from build123d import *

# Parameters (mm, degrees)
F0_R     = 4
F1_DEPTH = 3


with BuildPart() as f1:
    # F0 (on Front) → F1 (new body)
    with BuildSketch(Plane.XZ):
        with BuildLine():
            Line((53.104726, 7.336025), (-11.265956, 21.021994))
            ThreePointArc((-11.265956, 21.021994), (-14.82391, 21.160881), (-18.044949, 19.643238))
            Line((-18.044949, 19.643238), (-35.312375, 5.680292))
            ThreePointArc((-35.312375, 5.680292), (-37.891192, -0.597124), (-34.34867, -6.385628))
            Line((-34.34867, -6.385628), (-13.478804, -16.153186))
            ThreePointArc((-13.478804, -16.153186), (-11.393882, -16.717558), (-9.234581, -16.664338))
            Line((-9.234581, -16.664338), (52.653274, -7.417663))
            ThreePointArc((52.653274, -7.417663), (59.041491, -0.229387), (53.104726, 7.336025))
        make_face()
        with Locations((-30.415, 0)):
            Circle(F0_R, mode=Mode.SUBTRACT)
        with BuildLine():
            ThreePointArc((-15.273344, 12.239736), (-14.900729, 15.75558), (-11.384885, 15.382966))
            ThreePointArc((-11.384885, 15.382966), (-6.127117, 2.979875), (-8.230613, -10.326369))
            ThreePointArc((-8.230613, -10.326369), (-11.552104, -11.537854), (-12.76359, -8.216363))
            ThreePointArc((-12.76359, -8.216363), (-11.089905, 2.370991), (-15.273344, 12.239736))
        make_face(mode=Mode.SUBTRACT)
        with Locations((31.555, 0)):
            Circle(F0_R, mode=Mode.SUBTRACT)
        with Locations((51.545, 0)):
            Circle(F0_R, mode=Mode.SUBTRACT)
    extrude(amount=F1_DEPTH)


solid = f1.part
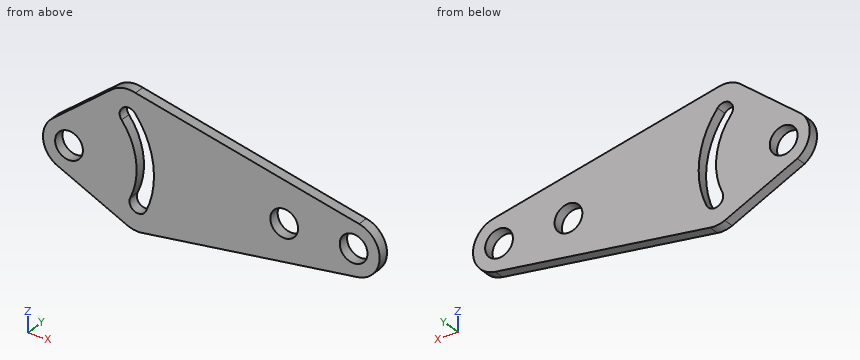
Verification items for the finished model (mm, model axes). Round coordinates to 2 decimals unless told otherwise and drop trailing zeros. Loops run counter-clockwise (first coordinate to the right, second up) from the corner with the lowest first, then second, coordinate; pieces in that order, holes last. Notation, with made-up numbers: (36.25, 85) - (90.25, 85) arc R18 cw to (90.25, 97) - close; hole circle Ø8 at (48, -1.5). An arc over 180 degrees is marked (long way). Answer in a Markdown table with one row per item. Add a question column.
Q1. Section check B-B on y = -0.7. Enter the section's corners in (x, z) (3 decimals), plus the area to 3 significant figures.
Q2. Material ranges on line 1 (X direction, y = -2.25, z = -2); line 2 (X direction, y = -2.8, z = 5); line 3 (Z direction, x = -27, y = -2.2), recorded low to high.
Q3. Gauge pin test, flat ends, axial feed: pin 1 (7 mm diameter, centred on x = 31.555, z = 0, fed in from +Y); pin 2 (1.5 mm diameter, centred on y = -2, z = -7.5, fed in from -X); pin 3 (1.5 mm diameter, centred on x = -10.5, y = -0.5, fed in from +Z); pin 4 (1 mm diameter, centred on y = -2.5, z = -3.5, fed in from -X). Record the tip position at first contact, or that the pin passes through.
Q4. Section check C-C on x = 39. Enter the section's corners in (y, z), plus the area to 3 significant figures.
Q5. Section check D-D on x = 4. Enter the section's corners in (y, z).
Q6. Section check A-A on z = 0. Enter the section's corners in (x, y) (3 decimals), plus the area to 3 significant figures.
Found:
| question | item | result |
|---|---|---|
| 1 | outline | (-35.312, 5.68) arc R7.5 ccw to (-34.349, -6.386) - (-13.479, -16.153) arc R7.5 ccw to (-9.235, -16.664) - (52.653, -7.418) arc R7.5 ccw to (53.105, 7.336) - (-11.266, 21.022) arc R7.5 ccw to (-18.045, 19.643) - close; hole circle Ø8 at (-30.415, 0); hole (-15.273, 12.24) arc R19.47 cw to (-12.764, -8.216) arc R2.5 ccw to (-8.231, -10.326) arc R24.47 ccw to (-11.385, 15.383) arc R2.5 ccw to start; hole circle Ø8 at (31.555, 0); hole circle Ø8 at (51.545, 0) |
| 1 | area | 2,130 mm² |
| 2 | line 1 | x = -37.64 to -33.88, -26.95 to -11.05, -6.03 to 28.09, 35.02 to 48.08, 55.01 to 58.77 |
| 2 | line 2 | x = -36.01 to -11.6, -6.46 to 57.14 |
| 2 | line 3 | z = -9.82 to -2.08, 2.08 to 12.4 |
| 3 | pin 1 | passes through |
| 3 | pin 2 | stops at x = -33.57 |
| 3 | pin 3 | stops at z = 21.02 |
| 3 | pin 4 | stops at x = -37.29 |
| 4 | outline | (-3, -9.46) - (0, -9.46) - (0, 10.33) - (-3, 10.33) - close |
| 4 | area | 59.4 mm² |
| 5 | outline | (-3, -14.69) - (0, -14.69) - (0, 17.78) - (-3, 17.78) - close |
| 6 | outline | (-37.915, -3) - (-34.415, -3) - (-34.415, 0) - (-37.915, 0) - close; (-26.415, -3) - (-10.945, -3) - (-10.945, 0) - (-26.415, 0) - close; (-5.945, -3) - (27.555, -3) - (27.555, 0) - (-5.945, 0) - close; (35.555, -3) - (47.545, -3) - (47.545, 0) - (35.555, 0) - close; (55.545, -3) - (59.045, -3) - (59.045, 0) - (55.545, 0) - close |
| 6 | area | 204 mm² |
